from build123d import *

# Parameters (mm, degrees)
F0_R     = 18.5674
F1_DEPTH = 10.922
F2_R     = 19.685
F3_DEPTH = 2.54
F4_SIZE  = 5.08
F5_R     = 0.508


with BuildPart() as f1:
    # F0 (on Top) → F1 (new body)
    with BuildSketch(Plane.XY):
        with BuildLine():
            Line((32.995568, -19.05), (0, 38.1))
            Line((0, 38.1), (-32.995568, -19.05))
            ThreePointArc((-32.995568, -19.05), (-31.954272, -20.749325), (-30.825541, -22.391874))
            Line((-30.825541, -22.391874), (30.825541, -22.391874))
            ThreePointArc((30.825541, -22.391874), (31.954272, -20.749325), (32.995568, -19.05))
        make_face()
        with Locations((0.09078, -2.456299)):
            Circle(F0_R, mode=Mode.SUBTRACT)
    extrude(amount=F1_DEPTH)

    # F2 (on Top) → F3 (join)
    with BuildSketch(Plane.XY):
        with Locations((0, -2.395251)):
            Circle(F2_R)
    extrude(amount=F3_DEPTH)

    # F4
    f4_edges = [f1.edges().sort_by_distance(p)[0] for p in [
        (0, 38.1, 5.461),
    ]]
    chamfer(f4_edges, length=F4_SIZE)

    # F5
    f5_edges = [f1.edges().sort_by_distance(p)[0] for p in [
        (17.767784, 7.325295, 10.922),
        (0, 33.700591, 10.922),
        (31.954272, -20.749325, 10.922),
        (-17.767784, 7.325295, 10.922),
        (0, -22.391874, 10.922),
        (-31.954272, -20.749325, 10.922),
        (-18.47662, -2.456299, 10.922),
        (17.767784, 7.325295, 0),
        (0, 33.700591, 0),
        (31.954272, -20.749325, 0),
        (-17.767784, 7.325295, 0),
        (0, -22.391874, 0),
        (-31.954272, -20.749325, 0),
    ]]
    fillet(f5_edges, radius=F5_R)


solid = f1.part
Check sheet for the modelled part. Datum: model origin and axes. Units: mm. A direction names the side the tool comes from. Give positions to 0.01 mm unless a question says otherwise; leave off trailing zeros. Loops run counter-clockwise (first coordinate to the right, second up) from the corner with the lowest first, then second, coordinate; pieces in that order, holes last. Notation, with made-up numbers: M 16.5,-26 L 23.5,-26 A3 cw 23.5,-21 Z; hole C -24.75,64 d2. An arc over 180 degrees is marked long. Use a Markdown table: item, result. Add a question column.
Q1. Tool access check on faces 1 (the flat face through (0, 33.701, 5)), 2 (the flat face through (0, -2, 2.54)). Record the directions out of +Z, -Z, +X, -X, +Y, -Y that give a thin tool (end or side, any length) a straight path to the whole face; none if there is none.
Q2. Go/stop test with flat-tipped pins: pin 1 (1.5 mm diameter, centred on x = 25.5, z = 3.5, fed in from +Y); pin 2 (5 mm diameter, centred on x = -6, z = 8, fed in from +Y); pin 3 (3 mm diameter, centred on x = 10.5, z = 1.5, fed in from +Y). Record where each tip stops, or that it passes through.
Q3. Sectioned sample at A-A, the plane z = 8. Record the cut outline in (x, y).
Q4. Scan lines: line 1 along Y through (x, z) = (0.5, 10); line 2 along X through (y, z) = (-10, 5.5); line 3 along Y through (x, z) = (-4, 10.25). Record each from-to range of solid material in increasing order. Write a range as [from, to].
Verdict:
| question | item | result |
|---|---|---|
| 1 | face 1 | +Z, -Z, +X, -X, +Y |
| 1 | face 2 | +Z |
| 2 | pin 1 | y = -4.77 |
| 2 | pin 2 | y = 32.04 |
| 2 | pin 3 | y = 22.51 |
| 3 | outline | M -33,-19.05 A38.1 ccw -30.83,-22.39 L 30.83,-22.39 A38.1 ccw 33,-19.05 L 2.54,33.7 L -2.54,33.7 Z; hole C 0.09,-2.46 d37.13 |
| 4 | line 1 | [-22.39, -21.02], [16.11, 33.7] |
| 4 | line 2 | [-27.77, -16.88], [17.06, 27.77] |
| 4 | line 3 | [-22.39, -20.57], [15.65, 31.17] |
